Study the drawing (mm; zero at the part's minimum x, y, z) and answer. Give positions to 0.01 mm unless a question says otherwise; leave off trailing zeros. Order: outer loops, then holes, each group sorted by start corner. A loop starts at its lowest first (then second) coordinate and runs counter-clockwise, first axis right, second up. Notation, with made-up numbers: (-31, 76.25) - (-14, 76.25) arc R15 ccw to (-14, 87.25) - close; hole circle Ø3 at (88.25, 83). An arc over 180 degrees is marked (long way). Return JSON: item names as keys, results as strings.
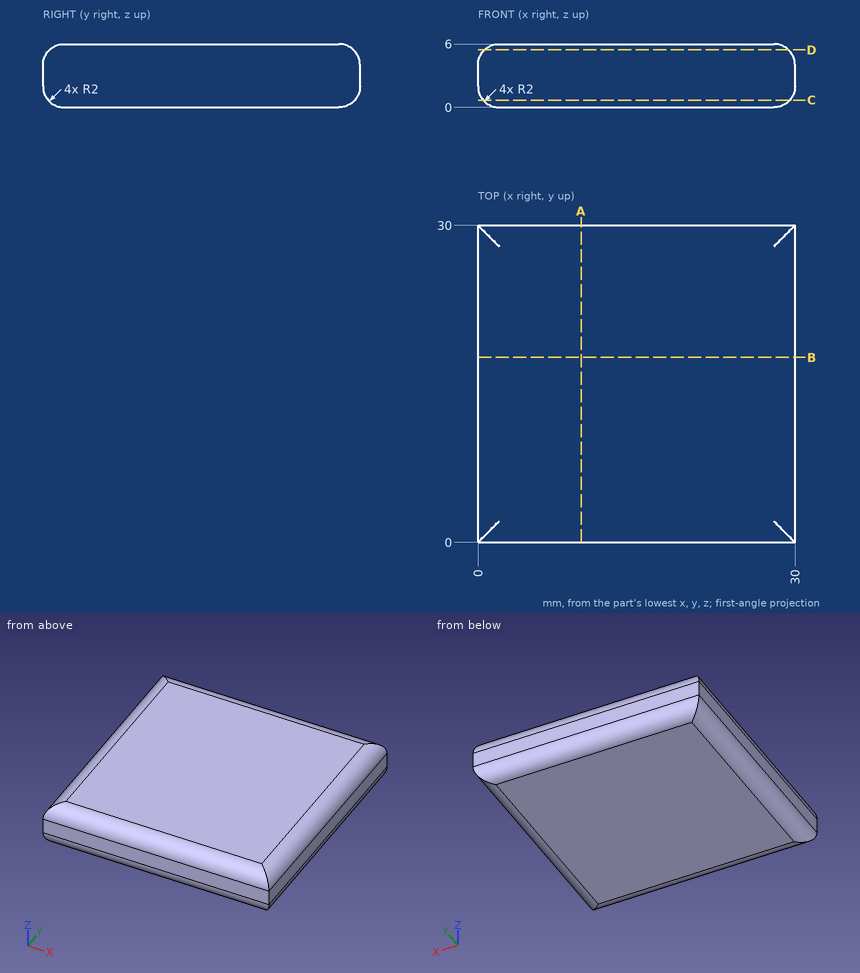
Q1. Given pin 1 (1 mm diameter, centred on y = 21, z = 5, fed in from +X), flat-ended and moving along its own axis, determine where the tip first touches the part or whether it passes through.
Values:
{"pin 1": "stops at x = 29.94"}
Q2. A cutting plane is placed at C-C (z = 0.7). Write down the section's boundary in (x, y), and give its area (3 significant figures).
Values:
{"outline": "(0.48, 0.48) - (29.52, 0.48) - (29.52, 29.52) - (0.48, 29.52) - close", "area": "843 mm²"}
Q3. A cutting plane is placed at D-D (z = 5.45). Write down the section's boundary in (x, y), and give its area (3 significant figures).
Values:
{"outline": "(0.62, 0.62) - (29.38, 0.62) - (29.38, 29.38) - (0.62, 29.38) - close", "area": "827 mm²"}
Q4. Consider L1, parallel to Y at x = 7.25, z = 1.5; L2, parallel to Y at x = 13, z = 1.2; L3, parallel to X at y = 18.25, z = 1.1. Determine where each line is inside the solid, lowest interval first.
Values:
{"L1": "y = 0.06 to 29.94", "L2": "y = 0.17 to 29.83", "L3": "x = 0.21 to 29.79"}
Q5. A cutting plane is placed at A-A (x = 9.75). Write down the section's boundary in (y, z).
Values:
{"outline": "(0, 2) arc R2 ccw to (2, 0) - (28, 0) arc R2 ccw to (30, 2) - (30, 4) arc R2 ccw to (28, 6) - (2, 6) arc R2 ccw to (0, 4) - close"}
